from build123d import *

# Parameters (mm, degrees)
F0_W     = 80
F0_H     = 80
F1_DEPTH = 20
F3_D     = 10
F3_DEPTH = 15
F3_TIP   = 3.0043030951
F5_DEPTH = 10
F6_DEPTH = 15


with BuildPart() as f1:
    # F0 (on Top) → F1 (new body)
    with BuildSketch(Plane.XY):
        Rectangle(F0_W, F0_H)
    extrude(amount=F1_DEPTH)

    # F3
    with Locations(Plane.XY.offset(20)):
        with Locations((-32, 20), (-32, -20)):
            Hole(F3_D / 2, depth=F3_DEPTH)
            with Locations((0, 0, -(F3_DEPTH + F3_TIP / 2))):  # 118° drill point
                Cone(0, F3_D / 2, F3_TIP, mode=Mode.SUBTRACT)

    # F4 (on face) → F5 (cut)
    with BuildSketch(Plane.XY.offset(20)):
        with BuildLine():
            Line((25, 35), (-15, 35))
            ThreePointArc((-15, 35), (-22.0710678119, 32.0710678119), (-25, 25))
            Line((-25, 25), (-25, -15))
            ThreePointArc((-25, -15), (-22.0710678119, -22.0710678119), (-15, -25))
            Line((-15, -25), (25, -25))
            ThreePointArc((25, -25), (32.0710678119, -22.0710678119), (35, -15))
            Line((35, -15), (35, 25))
            ThreePointArc((35, 25), (32.0710678119, 32.0710678119), (25, 35))
        make_face()
        with BuildLine():
            ThreePointArc((-15, 19), (-13.2426406871, 23.2426406871), (-9, 25))
            Line((-9, 25), (19, 25))
            ThreePointArc((19, 25), (23.2426406871, 23.2426406871), (25, 19))
            Line((25, 19), (25, -9))
            ThreePointArc((25, -9), (23.2426406871, -13.2426406871), (19, -15))
            Line((19, -15), (-9, -15))
            ThreePointArc((-9, -15), (-13.2426406871, -13.2426406871), (-15, -9))
            Line((-15, -9), (-15, 19))
        make_face(mode=Mode.SUBTRACT)
    extrude(amount=-F5_DEPTH, mode=Mode.SUBTRACT)

    # F6 (cut): a face of the model
    f6_faces = [f1.faces().sort_by_distance(p)[0] for p in [
        (5, 5, 20),
    ]]
    extrude(f6_faces, amount=-F6_DEPTH, mode=Mode.SUBTRACT)


solid = f1.part
Verification items for the finished model (mm, model axes). A direction names the side the tool comes from. Give positions to 0.01 mm unless a question says otherwise; leave off trailing zeros. Write each loop counter-clockwise with the first axis right and the second up, starting at its lowest first coordinate (ties: lowest second). Pieces come first, ordered by that corner, then holes.
(1) Material ranges on line 1 (X direction, y = 20, z = 14.25); line 2 (Y direction, x = -32, z = 14); line 3 (X direction, y = -16, z = 11.75), recorded low to high.
(2) Cross-section at C-C (y = 33.5). Enter the section's corners in (x, z).
(3) Cross-section at D-D (x = -11.5). Enter the section's corners in (y, z).
(4) Cross-section at B-B (x = 7.5). Enter the section's corners in (y, z), plus the area to 3 significant figures.
(5) Access from +Z, -Z, +X, -X, +Y, -Y to the whole of each face (thin tool, end or side, straight path). Record for faces 4 (the face through (-21.99, 32.15, 15.07)), 5 (the face through (-27, -8, 20)).
(6) Gauge pin test, flat ends, axial feed: pin 1 (6 mm diameter, centred on x = -32, y = -20, fed in from -Z); pin 2 (9 mm diameter, centred on x = -32, y = 20, fed in from +Z); pin 3 (12 mm diameter, centred on x = 10, y = 10, fed in from +Z). Record the tip position at first contact, or that the pin passes through.
(7) Mould release check, pull along Y, two halves, no side actions. Record for faces 1 (the face through (-1, 1, 0)), 2 (the face through (-13.289, 23.196, 7.535)), 3 (the face through (-1, 40, 10)): +Y half, -Y half, draft (parallel to the pull), parting line (faces both ways), or undercut.
(8) Cross-section at A-A (z = 9). Enter the section's corners in (x, y), plus the area to 3 significant figures.
Worked out:
1. line 1: x = -40 to -37, -27 to -25, 35 to 40
1. line 2: y = -40 to -25, -15 to 15, 25 to 40
1. line 3: x = -40 to -35, -29 to -24.95, 34.95 to 40
2. outline: (-40, 0) - (40, 0) - (40, 20) - (30.27, 20) - (30.27, 10) - (-20.27, 10) - (-20.27, 20) - (-40, 20) - close
3. outline: (-40, 0) - (40, 0) - (40, 20) - (35, 20) - (35, 10) - (24.45, 10) - (24.45, 5) - (-14.45, 5) - (-14.45, 10) - (-25, 10) - (-25, 20) - (-40, 20) - close
4. outline: (-40, 0) - (40, 0) - (40, 20) - (35, 20) - (35, 10) - (25, 10) - (25, 5) - (-15, 5) - (-15, 10) - (-25, 10) - (-25, 20) - (-40, 20) - close
4. area: 800 mm2
5. face 4: +Z
5. face 5: +Z, +X, -X, +Y, -Y
6. pin 1: stops at z = 0
6. pin 2: stops at z = 4.7
6. pin 3: stops at z = 5
7. face 1: draft
7. face 2: undercut
7. face 3: +Y half
8. outline: (-40, -40) - (40, -40) - (40, 40) - (-40, 40) - close; hole circle Ø10 at (-32, -20); hole circle Ø10 at (-32, 20); hole (-15, -9) arc R6 ccw to (-9, -15) - (19, -15) arc R6 ccw to (25, -9) - (25, 19) arc R6 ccw to (19, 25) - (-9, 25) arc R6 ccw to (-15, 19) - close
8. area: 4,670 mm2
